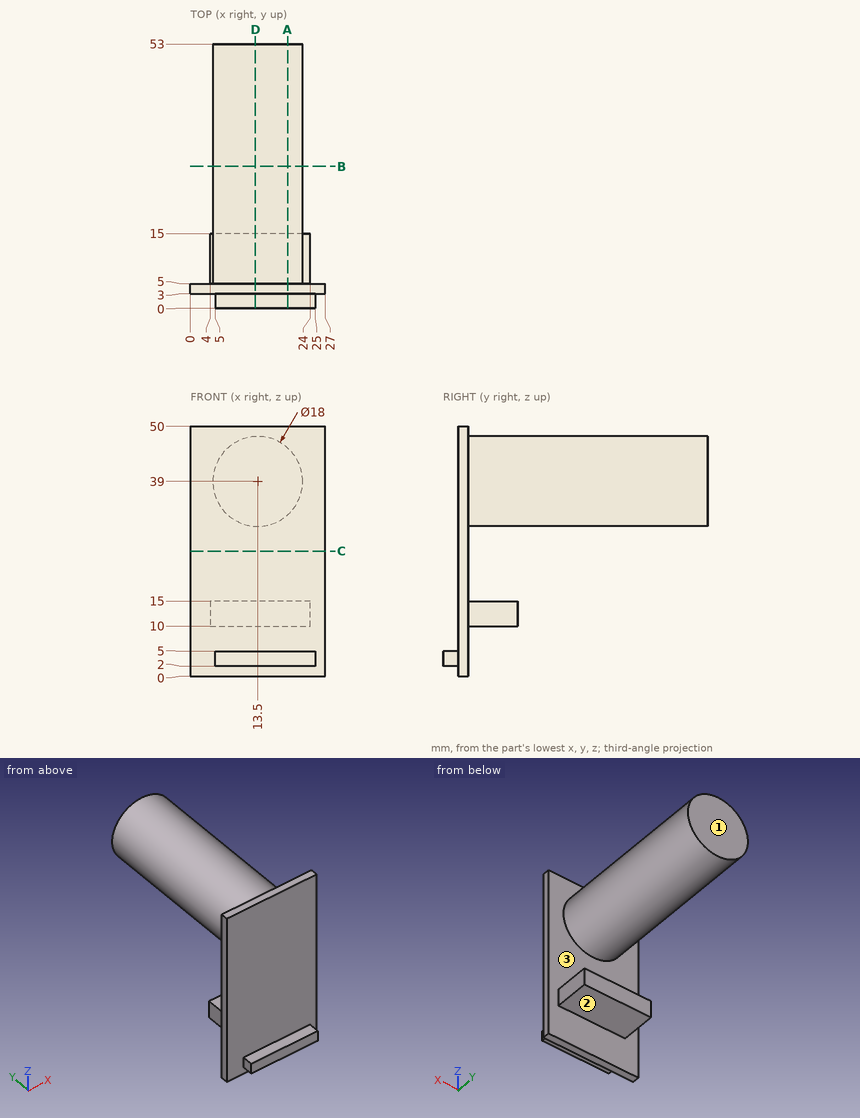
The drawing under review shows one solid part. Ordinate dimensions are in mm from its lowest x, y, z. Round coordinates to 2 decimals unless told otherwise and drop trailing zeros. Loops run counter-clockwise (first coordinate to the right, second up) from the corner with the lowest first, then second, coordinate; pieces in that order, holes last. Notation, with made-up numbers: (-9, 46.5) - (22, 46.5) arc R29 ccw to (22, 69.5) - close; hole circle Ø7 at (76, 62). An arc over 180 degrees is marked (long way). One line per question, with ' | ' between items.
1. Clearance check with flat-ended pins moving along their axes: P1, Ø8, axis at x = 16.5, z = 16, coming from the -Y side; P2, Ø1.5, axis at x = 15, y = 24, coming from the -Z side; P3, Ø4, axis at x = 9.5, z = 12, coming from the +Y side. State where each tip first meets the part, or that it passes through.
Results are:
P1: stops at y = 3 | P2: stops at z = 30.03 | P3: stops at y = 15
2. We need section D-D, the plane x = 13. State the section outline as (y, z) points, and give its area (3 significant figures).
Results are:
outline: (0, 2) - (3, 2) - (3, 0) - (5, 0) - (5, 10) - (15, 10) - (15, 15) - (5, 15) - (5, 30.01) - (53, 30.01) - (53, 47.99) - (5, 47.99) - (5, 50) - (3, 50) - (3, 5) - (0, 5) - close | area: 1,020 mm²
3. We need section A-A, the plane x = 19.5. State the section outline as (y, z) points.
Results are:
outline: (0, 2) - (3, 2) - (3, 0) - (5, 0) - (5, 10) - (15, 10) - (15, 15) - (5, 15) - (5, 32.29) - (53, 32.29) - (53, 45.71) - (5, 45.71) - (5, 50) - (3, 50) - (3, 5) - (0, 5) - close
4. Draft analysis for pull direction Z (two halves, no side actions). For the marked faces 1, 2 and 3, state which applies: released by +Z, released by -Z, zero draft, split by the parting line, or undercut.
Results are:
face 1: zero draft | face 2: released by -Z | face 3: undercut
5. For L1, parallel to Y at x = 12.5, z = 11; L2, parallel to Z at x = 13, y = 8.5; L3, parallel to X at y = 24.5, z = 39.5, list the stretches that pass through material, from the lowest coordinate up. Write a range as [from, to].
Results are:
L1: y = [3, 15] | L2: z = [10, 15], [30.01, 47.99] | L3: x = [4.51, 22.49]
6. We need section C-C, the plane z = 25. State the section outline as (x, y) points.
Results are:
outline: (0, 3) - (27, 3) - (27, 5) - (0, 5) - close
7. We need section B-B, the plane y = 28.5. State the section outline as (x, z) points.
Results are:
outline: circle Ø18 at (13.5, 39)
